Source: CAD feature listing. Evaluate the final solid. Frame: model axes, mm. Give positions to 0.01 mm unless a question says otherwise; leave off trailing zeros. Write each loop counter-clockwise with the first axis right and the second up, starting at its lowest first coordinate (ties: lowest second). Pieces come first, ordered by that corner, then holes.
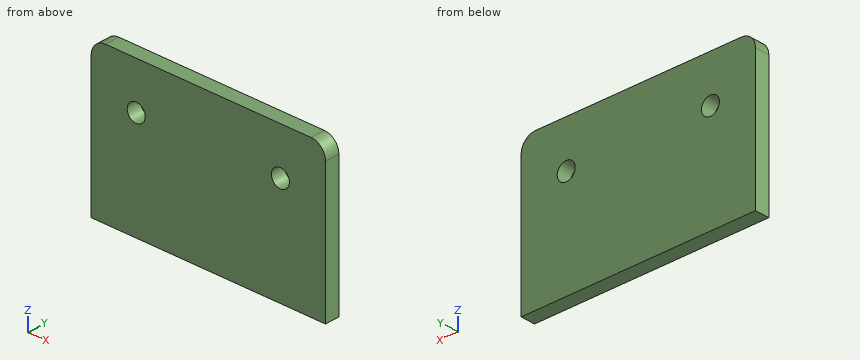
```python
from build123d import *

# Parameters (mm, degrees)
SKETCH1_R           = 2.5
BOSS_EXTRUDE1_DEPTH = 4


with BuildPart() as part:
    # Sketch1 → Boss-Extrude1 (new body)
    with BuildSketch(Plane(origin=(0, 0, 0), x_dir=(1, 0, 0), z_dir=(0, 1, 0))):
        with BuildLine():
            Line((4, 0), (61, 0))
            ThreePointArc((61, 0), (63.828427125, 1.171572875), (65, 4))
            Line((65, 4), (65, 42))
            Line((65, 42), (0, 42))
            Line((0, 42), (0, 4))
            ThreePointArc((0, 4), (1.171572875, 1.171572875), (4, 0))
        make_face()
        with Locations(Location((12.5, 12.75, 0), (0, 0, 270))):
            Circle(SKETCH1_R, mode=Mode.SUBTRACT)
        with Locations(Location((52.5, 12.75, 0), (0, 0, 270))):
            Circle(SKETCH1_R, mode=Mode.SUBTRACT)
    extrude(amount=BOSS_EXTRUDE1_DEPTH)


solid = part.part
```
1. Cut plane D-D, the plane x = 51. Return the cut outline in (y, z).
2. Contact query for a flat-ended pin moving along its axis: P1, Ø4, axis at x = 12.5, z = -12.75, coming from the +Y side. Output: stop coordinate, or through.
3. Line query: L1, parallel to X at y = 1.4, z = -12.75; L2, parallel to X at y = 3.65, z = -11; L3, parallel to Z at x = 3, y = 0.6. Output: solid intervals per line, ascending.
4. Cut plane C-C, the plane y = 2.3. Return the cut outline in (x, z).
5. Cut plane A-A, the plane z = -12.75. Return the cut outline in (x, y).
6. Cut plane B-B, the plane x = 12.5. Return the cut outline in (y, z).
Response values:
1. outline: (0, -42) - (4, -42) - (4, -14.75) - (0, -14.75) - close; (0, -10.75) - (4, -10.75) - (4, 0) - (0, 0) - close
2. P1: passes through
3. L1: x = 0 to 10, 15 to 50, 55 to 65
3. L2: x = 0 to 10.71, 14.29 to 50.71, 54.29 to 65
3. L3: z = -42 to -0.13
4. outline: (0, -42) - (65, -42) - (65, -4) arc R4 ccw to (61, 0) - (4, 0) arc R4 ccw to (0, -4) - close; hole circle Ø5 at (12.5, -12.75); hole circle Ø5 at (52.5, -12.75)
5. outline: (0, 0) - (10, 0) - (10, 4) - (0, 4) - close; (15, 0) - (50, 0) - (50, 4) - (15, 4) - close; (55, 0) - (65, 0) - (65, 4) - (55, 4) - close
6. outline: (0, -42) - (4, -42) - (4, -15.25) - (0, -15.25) - close; (0, -10.25) - (4, -10.25) - (4, 0) - (0, 0) - close
